Build history of the part. All positions in model axes, mm. Face numbers are marked on the shaded views. Coordinates: 2 decimals unless noted, no trailing zeros. Order: outer loops, then holes, each group sorted by start corner. A loop starts at its lowest first (then second) coordinate and runs counter-clockwise, first axis right, second up. Notation, with made-up numbers: (-19, 4.5) -> (-2, 4.5) arc R23 cw to (-2, 18.5) -> close; hole circle Ø6 at (13.5, -22.75). An arc over 180 degrees is marked (long way). Write each question's results on one line, items separated by ' | '.
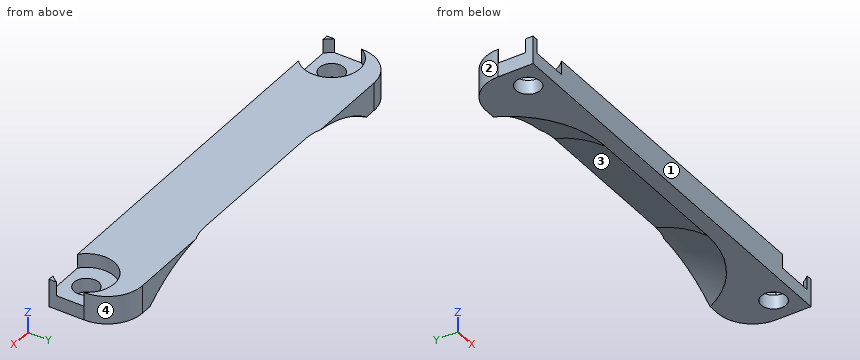
from build123d import *

# Parameters (mm, degrees)
SKETCH1_W           = 60
SKETCH1_H           = 10
BOSS_EXTRUDE1_DEPTH = 20.5
SKETCH3_W           = 60
SKETCH3_H           = 37
CUT_EXTRUDE1_DEPTH  = 38.686204372
FILLET1_R           = 5
SKETCH4_R           = 1.75
CUT_EXTRUDE2_DEPTH  = 31.6757233
SKETCH5_R           = 4
CUT_EXTRUDE5_DEPTH  = 2


with BuildPart() as part:
    # Sketch1 → Boss-Extrude1 (new, symmetric)
    with BuildSketch(Plane.XY):
        Rectangle(SKETCH1_W, SKETCH1_H)
    extrude(amount=BOSS_EXTRUDE1_DEPTH, both=True)

    # Sketch2 → Cut-Revolve1 (revolve, cut)
    with BuildSketch(Plane.XY):
        with BuildLine():
            Line((-32.5, 11), (32.5, 11))
            ThreePointArc((32.5, 11), (26.202795796, -4.202795796), (11, -10.5))
            Line((11, -10.5), (-11, -10.5))
            ThreePointArc((-11, -10.5), (-26.202795796, -4.202795796), (-32.5, 11))
        make_face()
    revolve(axis=Axis((-32.5, 11, 0), (1, 0, 0)), mode=Mode.SUBTRACT)

    # Sketch3 → Cut-Extrude1 (cut, through all)
    with BuildSketch(Plane(origin=(0, 5, 0), x_dir=(1, 0, 0), z_dir=(0, 1, 0))):
        with Locations((0, 2)):
            Rectangle(SKETCH3_W, SKETCH3_H)
    extrude(amount=-CUT_EXTRUDE1_DEPTH, mode=Mode.SUBTRACT)

    # Fillet1
    fillet1_edges = [part.edges().sort_by_distance(p)[0] for p in [
        (-30, 5, 18.5),
        (30, 5, 18.5),
    ]]
    fillet(fillet1_edges, radius=FILLET1_R)

    # Sketch4 → Cut-Extrude2 (cut, through all)
    with BuildSketch(Plane.XY.offset(20.5)):
        with Locations((-26.5, -2)):
            Circle(SKETCH4_R)
        with Locations((26.5, -2)):
            Circle(SKETCH4_R)
    extrude(amount=-CUT_EXTRUDE2_DEPTH, mode=Mode.SUBTRACT)

    # Sketch5 → Cut-Extrude5 (cut)
    with BuildSketch(Plane.XY.offset(20.5)):
        with Locations((-26.5, -2)):
            Circle(SKETCH5_R)
        with Locations((26.5, -2)):
            Circle(SKETCH5_R)
    extrude(amount=-CUT_EXTRUDE5_DEPTH, mode=Mode.SUBTRACT)


solid = part.part
Item 1: Slice it at D-D, the plane y = 0.5. List the corners of the cut face in (x, z).
Answer:
outline: (-29.97, 16.5) -> (-19.93, 16.5) arc R18.76 cw to (-11, 18.76) -> (11, 18.76) arc R18.76 cw to (19.93, 16.5) -> (29.97, 16.5) -> (29.97, 20.5) -> (29.62, 20.5) -> (29.62, 18.5) -> (23.38, 18.5) -> (23.38, 20.5) -> (-23.38, 20.5) -> (-23.38, 18.5) -> (-29.62, 18.5) -> (-29.62, 20.5) -> (-29.97, 20.5) -> close
Item 2: Pull direction X, two halves, no side cores. Call the marked faces 1, 2, 3 and 4: released by +X, released by -X, zero draft, split by the parting line, or undercut.
Answer:
face 1: zero draft | face 2: released by -X | face 3: undercut | face 4: released by +X
Item 3: Slice it at B-B, the plane x = 26. List the corners of the cut face in (y, z).
Answer:
outline: (-5, 16.5) -> (-3.68, 16.5) -> (-3.68, 18.5) -> (-5, 18.5) -> close; (-0.32, 16.5) -> (4.9, 16.5) -> (4.9, 20.5) -> (1.97, 20.5) -> (1.97, 18.5) -> (-0.32, 18.5) -> close
Item 4: Pin check, flat tip, straight feed: pin 1 (2 mm diameter, centred on x = -27, y = -0.5, fed in from +Z). Stop position of the tip, or through.
Answer:
pin 1: stops at z = 18.5
Item 5: Drill centre lines: line 1 (X direction, y = -3.5, z = 18.1); line 2 (X direction, y = -2, z = 19.2); line 3 (X direction, y = 3.25, z = 17.1). Where is each one in solid material? Low to high. Write a range as from..to.
Answer:
line 1: x = -30..-27.4, -25.6..25.6, 27.4..30 | line 2: x = -22.5..22.5 | line 3: x = -28.8..-21.48, 21.48..28.8
Item 6: Slice it at A-A, the plane z = 19.4. List the corners of the cut face in (x, y).
Answer:
outline: (-30, -5) -> (-29.15, -5) arc R4 cw to (-30, -3.94) -> close; (-30, -0.06) arc R4 cw (long way) to (-23.85, -5) -> (23.85, -5) arc R4 cw (long way) to (30, -0.06) -> (30, 0) arc R5 ccw to (25, 5) -> (18.06, 5) arc R9.27 cw to (11, 1.73) -> (-11, 1.73) arc R9.27 cw to (-18.06, 5) -> (-25, 5) arc R5 ccw to (-30, 0) -> close; (29.15, -5) -> (30, -5) -> (30, -3.94) arc R4 cw to start
Item 7: Slice it at C-C, the plane y = -2. List the corners of the cut face in (x, z), and give its area (3 significant figures).
Answer:
outline: (-30, 16.5) -> (-28.25, 16.5) -> (-28.25, 18.5) -> (-30, 18.5) -> close; (-24.75, 16.5) -> (-15.58, 16.5) arc R17.12 cw to (-11, 17.12) -> (11, 17.12) arc R17.12 cw to (15.58, 16.5) -> (24.75, 16.5) -> (24.75, 18.5) -> (22.5, 18.5) -> (22.5, 20.5) -> (-22.5, 20.5) -> (-22.5, 18.5) -> (-24.75, 18.5) -> close; (28.25, 16.5) -> (30, 16.5) -> (30, 18.5) -> (28.25, 18.5) -> close | area: 178 mm^2
